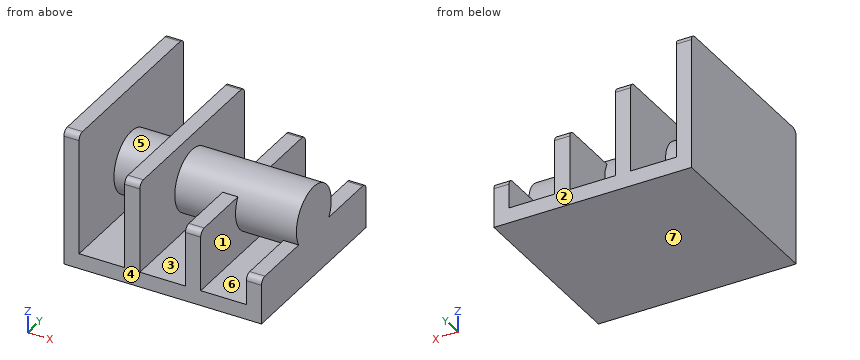
from build123d import *

# Parameters (mm, degrees)
F0_W     = 12.7
F0_H     = 76.2
F0_H_2   = 50.8
F1_DEPTH = 152.4
F2_R     = 25.4
F3_DEPTH = 165.1
F4_R     = 5.08


with BuildPart() as f1:
    # F0 (on Front) → F1 (new body)
    with BuildSketch(Plane.XZ):
        Polygon((-50.8, 93.861793), (-63.5, 93.861793), (-63.5, -20.438207), (101.6, -20.438207), (101.6, 17.661793), (88.9, 17.661793), (88.9, -7.738207), (50.8, -7.738207), (38.1, -7.738207), (32.964252, -7.738207), (0, -7.738207), (-12.7, -7.738207), (-50.8, -7.738207), align=None)
        with Locations((-6.35, 30.361793)):
            Rectangle(F0_W, F0_H)
        with Locations((44.45, 17.661793)):
            Rectangle(F0_W, F0_H_2)
    extrude(amount=F1_DEPTH)

    # F2 (on face) → F3 (join)
    with BuildSketch(Plane(origin=(-63.5, 0, 0), x_dir=(0, -1, 0), z_dir=(-1, 0, 0))):
        with Locations((76.2, 30.361793)):
            Circle(F2_R)
    extrude(amount=-F3_DEPTH)

    # F4
    f4_edges = [f1.edges().sort_by_distance(p)[0] for p in [
        (-57.15, -152.4, 93.861793),
        (-57.15, 0, 93.861793),
        (-6.35, -152.4, 68.461793),
        (-6.35, 0, 68.461793),
        (44.45, 0, 43.061793),
        (44.45, -152.4, 43.061793),
        (95.25, -152.4, 17.661793),
        (95.25, 0, 17.661793),
    ]]
    fillet(f4_edges, radius=F4_R)


solid = f1.part
Read the model definition and answer for the solid it produces. Units are mm, in the model's axes. Face numbers are marked on the shaded views. A direction names the side the tool comes from. Give positions to 0.01 mm unless a question says otherwise; leave off trailing zeros. Write each loop counter-clockwise with the first axis right and the second up, starting at its lowest first coordinate (ties: lowest second). Pieces come first, ordered by that corner, then holes. Notation, with made-up numbers: M 42,57 L 71,57 A16 ccw 71,72 Z; hole C -28.75,85.25 d8. An arc over 180 degrees is marked long. One line per item, written item: value. Start each with the question number.
(1) Determine the mould class of the marked faces 4, 5, 6 and 7 for opening direction Z: pulls with the +Z half, pulls with the -Z half, needs draft (parallel to the pull), parting line crosses it, or undercut.
(2) Find section A-A (y = -76.2). Determine the outline of the cut face in (x, z), plus the area to 3 significant figures.
(3) Find section D-D (z = 33). Determine the outline of the cut face in (x, y).
(4) Find the intervals of material crossed by line 1 (X direction, y = -26.5, z = 36); line 2 (X direction, y = -111, z = -3); line 3 (X direction, y = -6.5, z = 60.5), in increasing order.
(5) Find section B-B (y = -134). Determine the outline of the cut face in (x, z), plus the area to 3 significant figures.
(6) Flat-ended cylindrical pins translate along their axes: pin 1 Ø2 at (x, y) = (-7.5, -133) entering from +Z; pin 2 Ø8 at (x, y) = (-45, -40.5) entering from +Z; pin 3 Ø11.5 at (x, y) = (76.5, -75.5) entering from +Z. Find the tip coordinate at first contact, or state that the pin passes through.
(7) Find section C-C (x = 12.5). Determine the outline of the cut face in (y, z).
(8) A tool of negligible diameter and unlimited length cuts with its end or side. For the marked faces 1, 2 and 3, from which of +Z, -Z, +X, -X, +Y, -Y can it reach the whole face along a straight path? Write none if from no direction.
Results below:
1. face 4: needs draft
1. face 5: undercut
1. face 6: undercut
1. face 7: pulls with the -Z half
2. outline: M -63.5,-20.44 L 101.6,-20.44 L 101.6,55.76 L 0,55.76 L 0,68.46 L -12.7,68.46 L -12.7,55.76 L -50.8,55.76 L -50.8,93.86 L -63.5,93.86 Z; hole M -50.8,-7.74 L -12.7,-7.74 L -12.7,4.96 L -50.8,4.96 Z; hole M 0,-7.74 L 38.1,-7.74 L 38.1,4.96 L 0,4.96 Z; hole M 50.8,-7.74 L 88.9,-7.74 L 88.9,4.96 L 50.8,4.96 Z
2. area: 11,800 mm^2
3. outline: M -63.5,-152.4 L -50.8,-152.4 L -50.8,-101.46 L -12.7,-101.46 L -12.7,-152.4 L 0,-152.4 L 0,-101.46 L 38.1,-101.46 L 38.1,-152.4 L 50.8,-152.4 L 50.8,-101.46 L 101.6,-101.46 L 101.6,-50.94 L 50.8,-50.94 L 50.8,0 L 38.1,0 L 38.1,-50.94 L 0,-50.94 L 0,0 L -12.7,0 L -12.7,-50.94 L -50.8,-50.94 L -50.8,0 L -63.5,0 Z
4. line 1: x = -63.5 to -50.8, -12.7 to 0, 38.1 to 50.8
4. line 2: x = -63.5 to -50.8, -12.7 to 0, 38.1 to 50.8, 88.9 to 101.6
4. line 3: x = -63.5 to -50.8, -12.7 to 0
5. outline: M -63.5,-20.44 L 101.6,-20.44 L 101.6,17.66 L 88.9,17.66 L 88.9,-7.74 L 50.8,-7.74 L 50.8,43.06 L 38.1,43.06 L 38.1,-7.74 L 0,-7.74 L 0,68.46 L -12.7,68.46 L -12.7,-7.74 L -50.8,-7.74 L -50.8,93.86 L -63.5,93.86 Z
5. area: 5,320 mm^2
6. pin 1: stops at z = 68.46
6. pin 2: stops at z = -7.74
6. pin 3: stops at z = 55.76
7. outline: M -152.4,-20.44 L 0,-20.44 L 0,-7.74 L -152.4,-7.74 Z; C -76.2,30.36 d50.8
8. face 1: none
8. face 2: +Z, -Z, +X, -X, +Y
8. face 3: +Y, -Y
